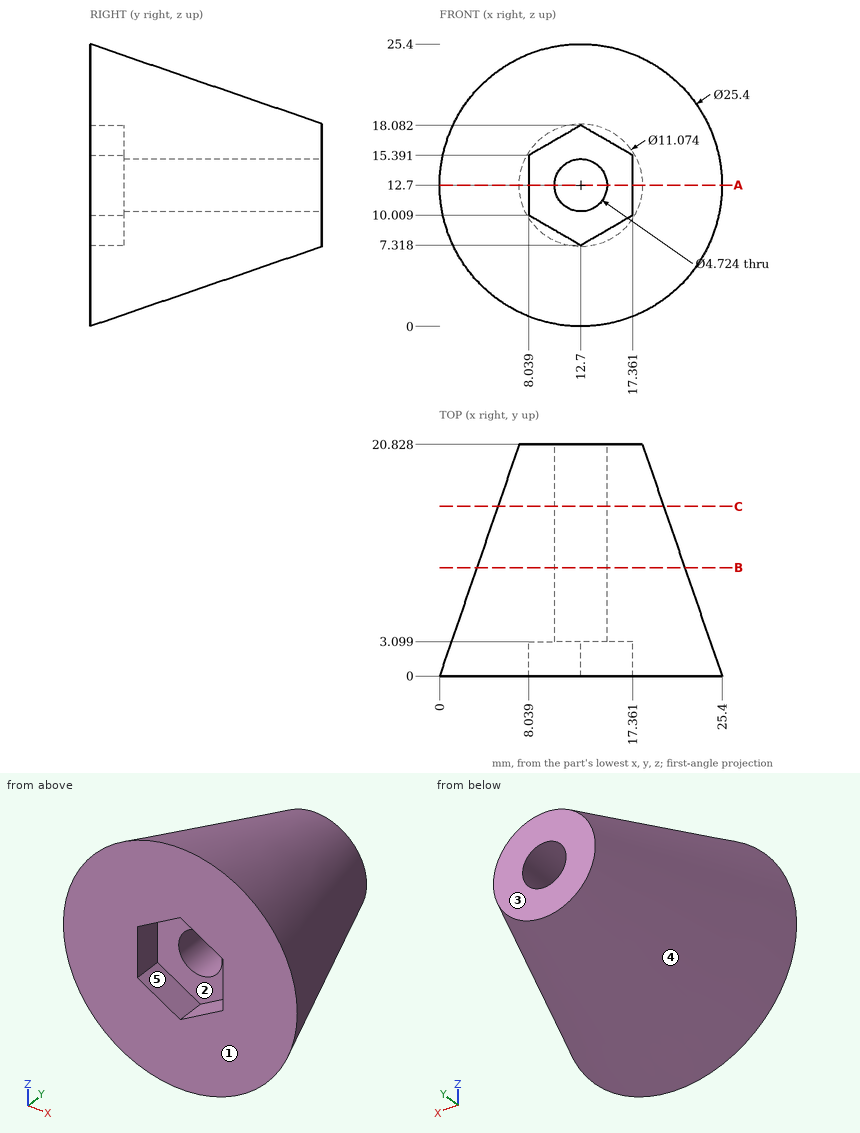
Drawing for the job (mm, zero at the part's lowest x, y, z). A direction names the side the tool comes from. Coordinates: 2 decimals unless noted, no trailing zeros. Write each loop counter-clockwise with the first axis right and the second up, starting at its lowest first coordinate (ties: lowest second). Pieces come first, ordered by that corner, then holes. Notation, with made-up numbers: (40.5, -21) -> (74.5, -21) arc R21 cw to (74.5, 18) -> close; hole circle Ø5 at (66, 54.25). An arc over 180 degrees is marked (long way). One line per item, written item: value. Start each with the question number.
1) Probe probe 1 along X at (y, z) = (12.5, 12.7); probe 2 along Z at (x, y) = (14.75, 9.75) (1 decimal); probe 3 along Y at (x, z) = (9.25, 13.75). List the from-to ranges inside material, lowest first.
2) Slice it at A-A on z = 12.7. Write the cut outline in (x, y), then the cut area to 3 significant figures.
3) Pull direction X, two halves, no side cores. Call the marked faces 3, 4 and 5: +X half, -X half, draft (parallel to the pull), parting line (faces both ways), or undercut.
4) Which spindle directions (+Z, -Z, +X, -X, +Y, -Y) get a long thin tool onto all of the face, cutting with end or side? Do the marked faces 1 and 2. Say none if no direction does.
5) Flat gauge pins, fed straight in: pin 1 Ø4 at (x, y) = (16, 13.5) entering from -Z; pin 2 Ø3 at (x, y) = (20.5, 3.5) entering from -Z; pin 3 Ø10 at (y, z) = (3, 4) entering from -X; pin 4 Ø2.5 at (y, z) = (1, 13) entering from +X. Where does each tip first touch, or does it go through?
6) Slice it at B-B on y = 9.75. Write the cut outline in (x, z) (1 decimal).
7) Slice it at C-C on y = 15.25. Write the cut outline in (x, z) (1 decimal), then the cut area to 3 significant figures.
Answers follow:
1. probe 1: 4.3 to 10.34, 15.06 to 21.1
1. probe 2: 3.6 to 11.5, 13.9 to 21.8
1. probe 3: 3.1 to 20.83
2. outline: (0, 0) -> (8.04, 0) -> (8.04, 3.1) -> (10.34, 3.1) -> (10.34, 20.83) -> (7.16, 20.83) -> close; (15.06, 3.1) -> (17.36, 3.1) -> (17.36, 0) -> (25.4, 0) -> (18.24, 20.83) -> (15.06, 20.83) -> close
2. area: 267 mm2
3. face 3: draft
3. face 4: parting line
3. face 5: undercut
4. face 1: +Z, -Z, +X, -X, -Y
4. face 2: -Y
5. pin 1: z = 4.35
5. pin 2: z = 2.91
5. pin 3: x = 0.9
5. pin 4: x = 25.4
6. outline: circle Ø18.7 at (12.7, 12.7); hole circle Ø4.7 at (12.7, 12.7)
7. outline: circle Ø14.9 at (12.7, 12.7); hole circle Ø4.7 at (12.7, 12.7)
7. area: 157 mm2
